```python
from build123d import *

# Parameters (mm, degrees)
BASE_FLANGE1_DEPTH = 80
CUT_EXTRUDE1_DEPTH = 158
SKETCH7_R          = 2.5
CUT_EXTRUDE2_DEPTH = 158


# Sheet-metal steps are written as plain solids
with BuildPart() as part:
    # Sketch1 → Base-Flange1 (new body)
    with BuildSketch(Plane.XY):
        with BuildLine():
            Line((0, 0), (-64, 0))
            ThreePointArc((-64, 0), (-68.242640687, 1.757359313), (-70, 6))
            Line((-70, 6), (-70, 64))
            ThreePointArc((-70, 64), (-68.242640687, 68.242640687), (-64, 70))
            Line((-64, 70), (0, 70))
            Line((0, 70), (0, 67))
            Line((0, 67), (-64, 67))
            ThreePointArc((-64, 67), (-66.121320344, 66.121320344), (-67, 64))
            Line((-67, 64), (-67, 6))
            ThreePointArc((-67, 6), (-66.121320344, 3.878679656), (-64, 3))
            Line((-64, 3), (0, 3))
            Line((0, 3), (0, 0))
        make_face()
    extrude(amount=BASE_FLANGE1_DEPTH)

    # Sketch6 → Cut-Extrude1 (cut)
    with BuildSketch(Plane.XZ):
        Polygon((0, 80), (-10, 80), (0, 30), align=None)
    extrude(amount=-CUT_EXTRUDE1_DEPTH, mode=Mode.SUBTRACT)

    # Sketch7 → Cut-Extrude2 (cut)
    with BuildSketch(Plane.XZ):
        with Locations(Location((-30, 50, 0), (0, 0, 270))):
            Circle(SKETCH7_R)
    extrude(amount=-CUT_EXTRUDE2_DEPTH, mode=Mode.SUBTRACT)


solid = part.part
```
Geometry: final body of the model. Coordinates: model frame, mm. A direction names the side the tool comes from. Give positions to 0.01 mm unless a question says otherwise; leave off trailing zeros. Loops run counter-clockwise (first coordinate to the right, second up) from the corner with the lowest first, then second, coordinate; pieces in that order, holes last. Notation, with made-up numbers: (23.25, 3.25) -> (33.25, 3.25) arc R26 cw to (33.25, 27.25) -> close; hole circle Ø1 at (-40, 78.25). An arc over 180 degrees is marked (long way). Use one line per item in the form item = value.
Item 1: Line query: probe 1 along Y at (x, z) = (-14, 20.5); probe 2 along Y at (x, z) = (-66, 34); probe 3 along X at (y, z) = (1, 50). Output: solid intervals per line, ascending.
A:
probe_1 = 0 to 3, 67 to 70
probe_2 = 0.34 to 3.76, 66.24 to 69.66
probe_3 = -67.32 to -32.5, -27.5 to -4
Item 2: Access query for faces 5 (the face through (-66.1, 66.14, 39.44)), 6 (the face through (-5, 68, 55)). Directions: +Z, -Z, +X, -X, +Y, -Y. A direction counts if a zero-diameter tool reaches every point of the face in a straight line with its end or side. Return the directions, or none.
A:
face_5 = +Z, -Z, +X
face_6 = +Z, +X, +Y, -Y
Item 3: Section query C-C on x = -38. Output: boundary loops of the cut face in (y, z), and give its area (3 significant figures).
A:
outline = (0, 0) -> (3, 0) -> (3, 80) -> (0, 80) -> close; (67, 0) -> (70, 0) -> (70, 80) -> (67, 80) -> close
area = 480 mm^2
Item 4: Section query B-B on z = 50. Output: boundary loops of the cut face in (x, y).
A:
outline = (-70, 6) arc R6 ccw to (-64, 0) -> (-32.5, 0) -> (-32.5, 3) -> (-64, 3) arc R3 cw to (-67, 6) -> (-67, 64) arc R3 cw to (-64, 67) -> (-32.5, 67) -> (-32.5, 70) -> (-64, 70) arc R6 ccw to (-70, 64) -> close; (-27.5, 0) -> (-4, 0) -> (-4, 3) -> (-27.5, 3) -> close; (-27.5, 67) -> (-4, 67) -> (-4, 70) -> (-27.5, 70) -> close
Item 5: Pin query (flat end, axial travel): P1, Ø6, axis at y = 54, z = 11, coming from the +X side; P2, Ø10, axis at y = 9.5, z = 50.5, coming from the +X side. Return the tip coordinate at first contact, or that it passes through.
A:
P1 = -67
P2 = -66.6
Item 6: Section query D-D on z = 39. Output: boundary loops of the cut face in (x, y), and give its area (3 significant figures).
A:
outline = (-70, 6) arc R6 ccw to (-64, 0) -> (-1.8, 0) -> (-1.8, 3) -> (-64, 3) arc R3 cw to (-67, 6) -> (-67, 64) arc R3 cw to (-64, 67) -> (-1.8, 67) -> (-1.8, 70) -> (-64, 70) arc R6 ccw to (-70, 64) -> close
area = 590 mm^2
Item 7: Section query A-A on x = -30. Output: boundary loops of the cut face in (y, z), and give its area (3 significant figures).
A:
outline = (0, 0) -> (3, 0) -> (3, 47.5) -> (0, 47.5) -> close; (0, 52.5) -> (3, 52.5) -> (3, 80) -> (0, 80) -> close; (67, 0) -> (70, 0) -> (70, 47.5) -> (67, 47.5) -> close; (67, 52.5) -> (70, 52.5) -> (70, 80) -> (67, 80) -> close
area = 450 mm^2
Item 8: Draft query along X for faces 1 (the face through (-32, 67, 39)), 2 (the face through (-27.89, 68.48, 48.66)), 3 (the face through (-27.89, 1.48, 48.66)), 4 (the face through (-67, 35, 39)). Return one class per face: pulls with the +X half, pulls with the -X half, needs draft (parallel to the pull), parting line crosses it, or undercut.
A:
face_1 = needs draft
face_2 = undercut
face_3 = undercut
face_4 = pulls with the +X half
